```python
from build123d import *

# Parameters (mm, degrees)
F0_R     = 15.86
F1_DEPTH = 4.45


with BuildPart() as f1:
    # F0 (on Top) → F1 (new body)
    with BuildSketch(Plane.XY):
        Polygon((33.6925, -33.5685), (50, -33.5685), (54.45, -33.5685), (54.45, -16.64242), (50, -16.64242), (50, 16.64242), (54.45, 16.64242), (54.45, 34.008425), (50, 34.008425), (50, 38.0185), (33.6925, 38.0185), (33.6925, 33.5685), (-33.6925, 33.5685), (-33.6925, 38.0185), (-50, 38.0185), (-50, 33.5685), (-50, 16.64242), (-54.45, 16.64242), (-54.45, -16.64242), (-50, -16.64242), (-50, -33.5685), (-33.6925, -33.5685), (-33.6925, -38.0185), (33.6925, -38.0185), align=None)
        with Locations((-22.039123, 0)):
            Circle(F0_R, mode=Mode.SUBTRACT)
        with Locations((22.039123, 0)):
            Circle(F0_R, mode=Mode.SUBTRACT)
    extrude(amount=F1_DEPTH)


solid = f1.part
```
Geometry check sheet. Reference: the model listing, model coordinates, mm. A direction names the side the tool comes from. Coordinates: 2 decimals unless noted, no trailing zeros. Write each loop counter-clockwise with the first axis right and the second up, starting at its lowest first coordinate (ties: lowest second). Pieces come first, ordered by that corner, then holes. Notation, with made-up numbers: M 23,73 L 42,73 A4 ccw 42,78 Z; hole C 52.25,77 d11. An arc over 180 degrees is marked long. Answer as a JSON object with one key per item and string values.
1. Section check B-B, the plane y = 0. Enter the section's corners in (x, z).
Answers below:
{"outline": "M -54.45,0 L -37.9,0 L -37.9,4.45 L -54.45,4.45 Z; M -6.18,0 L 6.18,0 L 6.18,4.45 L -6.18,4.45 Z; M 37.9,0 L 50,0 L 50,4.45 L 37.9,4.45 Z"}
2. Tool access check on faces 5 (the flat face through (0, 33.568, 2)), 6 (the flat face through (-50, 27, 2)), 7 (the flat face through (50, 36, 2)), 8 (the flat face through (-50, -25, 2)). Record the directions out of +Z, -Z, +X, -X, +Y, -Y that give a thin tool (end or side, any length) a straight path to the whole face; none if there is none.
Answers below:
{"face 5": "+Z, -Z, +Y", "face 6": "+Z, -Z, -X, +Y", "face 7": "+Z, -Z, +X, +Y", "face 8": "+Z, -Z, -X, -Y"}
3. Draft check along Y on faces 1 (the flat face through (-52, -16.642, 2)), 2 (the flat face through (33.692, 36, 2)), 3 (the flat face through (-42, 38.018, 2)), 4 (the flat face through (52, -16.642, 2)). Enter one of: released by +Y, released by -Y, zero draft, split by the parting line, or undercut.
Answers below:
{"face 1": "released by -Y", "face 2": "zero draft", "face 3": "released by +Y", "face 4": "undercut"}
4. Scan lines: L1, parallel to X at y = 4, z = 1.35; L2, parallel to X at y = 7, z = 2.65; L3, parallel to X at y = 33.5, z = 2.1. Record each from-to range of solid material in increasing order.
Answers below:
{"L1": "x = -54.45 to -37.39, -6.69 to 6.69, 37.39 to 50", "L2": "x = -54.45 to -36.27, -7.81 to 7.81, 36.27 to 50", "L3": "x = -50 to 54.45"}
5. Section check A-A, the plane z = 3.45. Enter the section's corners in (x, y).
Answers below:
{"outline": "M -54.45,-16.64 L -50,-16.64 L -50,-33.57 L -33.69,-33.57 L -33.69,-38.02 L 33.69,-38.02 L 33.69,-33.57 L 54.45,-33.57 L 54.45,-16.64 L 50,-16.64 L 50,16.64 L 54.45,16.64 L 54.45,34.01 L 50,34.01 L 50,38.02 L 33.69,38.02 L 33.69,33.57 L -33.69,33.57 L -33.69,38.02 L -50,38.02 L -50,16.64 L -54.45,16.64 Z; hole C -22.04,0 d31.72; hole C 22.04,0 d31.72"}
6. Go/stop test with flat-tipped pins: pin 1 Ø1.3 at (y, z) = (26.5, 1.5) entering from -X; pin 2 Ø2 at (x, z) = (-14.5, 2.5) entering from +Y; pin 3 Ø2 at (x, z) = (51.5, 3) entering from +Y; pin 4 Ø1.5 at (x, y) = (-0.5, 14.5) entering from -Z. Record where each tip stops, or that it passes through.
Answers below:
{"pin 1": "stops at x = -50", "pin 2": "stops at y = 33.57", "pin 3": "stops at y = 34.01", "pin 4": "stops at z = 0"}
7. Section check D-D, the plane y = -28. Enter the section's corners in (x, z), plus the area to 3 significant figures.
Answers below:
{"outline": "M -50,0 L 54.45,0 L 54.45,4.45 L -50,4.45 Z", "area": "465 mm²"}
8. Section check C-C, the plane x = 9. Enter the section's corners in (y, z), plus the area to 3 significant figures.
Answers below:
{"outline": "M -38.02,0 L -9.03,0 L -9.03,4.45 L -38.02,4.45 Z; M 9.03,0 L 33.57,0 L 33.57,4.45 L 9.03,4.45 Z", "area": "238 mm²"}
